Geometry check sheet. Reference: the model listing, model coordinates, mm. A direction names the side the tool comes from. Round coordinates to 2 decimals unless told otherwise and drop trailing zeros. Order: outer loops, then holes, each group sorted by start corner. A loop starts at its lowest first (then second) coordinate and runs counter-clockwise, first axis right, second up.
(1) Cross-section at A-A on x = 0. Enter the section's corners in (y, z) (1 decimal), and give its area (3 significant figures).
(2) Cross-section at B-B on z = 0. Enter the section's corners in (x, y) (1 decimal), and give its area (3 significant figures).
(3) Draft check along X on faces 3 (the face through (0, 29.21, 0)), 4 (the face through (1.93, 20.84, 2.52)), 5 (the face through (0, 3.175, 0)), 6 (the face through (-7.75, 1.57, 1.72)). Enter one of: pulls with the +X half, pulls with the -X half, needs draft (parallel to the pull), parting line crosses it, or undercut.
(4) Set-up check for faces 1 (the face through (-6, 10.16, 0)), 2 (the face through (8, 0, -2)): record each of +Z, -Z, +X, -X, +Y, -Y from which the full face is reachable in a straight line by a thin tool's end or side.
(5) Thickness scan on L1, parallel to X at y = 1.65, z = 0 (1 decimal); L2, parallel to Y at x = -2.5, z = 8.25; L3, parallel to Y at x = 5.75, z = -2 (3 decimals). Record the ranges inside material, lowest first.
(6) Cross-section at D-D on x = 7.5. Enter the section's corners in (y, z) (3 decimals), and give its area (3 significant figures).
(7) Cross-section at C-C on y = 6.5. Enter the section's corners in (x, z) (3 decimals), and give its area (3 significant figures).
(8) Gauge pin test, flat ends, axial feed: P1, Ø1.5, axis at y = 6.5, z = -2, coming from the +X side; P2, Ø5, axis at x = 3, z = 2, coming from the -Y side (3 decimals); P3, Ø6, axis at x = 3.5, y = 21.5, coming from the -Z side; P4, Ø3, axis at x = 6, y = 17.5, coming from the -Z side. Record the tip position at first contact, or that the pin passes through.
from build123d import *

# Parameters (mm, degrees)
SKETCH1_R           = 9.525
BOSS_EXTRUDE1_DEPTH = 10.16
SKETCH2_R           = 7.9375
CUT_EXTRUDE1_DEPTH  = 3.175
SKETCH3_R           = 3.175
BOSS_EXTRUDE2_DEPTH = 19.05
FILLET1_R           = 2.54


with BuildPart() as part:
    # Sketch1 → Boss-Extrude1 (new body)
    with BuildSketch(Plane(origin=(0, 0, 0), x_dir=(1, 0, 0), z_dir=(0, 1, 0))):
        with Locations(Location((0, 0, 0), (0, 0, 270))):
            Circle(SKETCH1_R)
    extrude(amount=BOSS_EXTRUDE1_DEPTH)

    # Sketch2 → Cut-Extrude1 (cut)
    with BuildSketch(Plane(origin=(0, 0, 0), x_dir=(-1, 0, 0), z_dir=(0, -1, 0))):
        with Locations(Location((0, 0, 0), (0, 0, 90))):
            Circle(SKETCH2_R)
    extrude(amount=-CUT_EXTRUDE1_DEPTH, mode=Mode.SUBTRACT)

    # Sketch3 → Boss-Extrude2 (add)
    with BuildSketch(Plane(origin=(0, 10.16, 0), x_dir=(1, 0, 0), z_dir=(0, 1, 0))):
        with Locations(Location((0, 0, 0), (0, 0, 90))):
            Circle(SKETCH3_R)
    extrude(amount=BOSS_EXTRUDE2_DEPTH)

    # Fillet1
    fillet1_edges = [part.edges().sort_by_distance(p)[0] for p in [
        (0, 10.16, 3.175),
    ]]
    fillet(fillet1_edges, radius=FILLET1_R)


solid = part.part
Found:
1. outline: (0, -9.5) - (10.2, -9.5) - (10.2, -5.7) arc R2.5 cw to (12.7, -3.2) - (29.2, -3.2) - (29.2, 3.2) - (12.7, 3.2) arc R2.5 cw to (10.2, 5.7) - (10.2, 9.5) - (0, 9.5) - (0, 7.9) - (3.2, 7.9) - (3.2, -7.9) - (0, -7.9) - close
1. area: 267 mm2
2. outline: (-9.5, 0) - (-7.9, 0) - (-7.9, 3.2) - (7.9, 3.2) - (7.9, 0) - (9.5, 0) - (9.5, 10.2) - (5.7, 10.2) arc R2.5 cw to (3.2, 12.7) - (3.2, 29.2) - (-3.2, 29.2) - (-3.2, 12.7) arc R2.5 cw to (-5.7, 10.2) - (-9.5, 10.2) - close
2. area: 267 mm2
3. face 3: needs draft
3. face 4: parting line crosses it
3. face 5: undercut
3. face 6: undercut
4. face 1: +Y
4. face 2: +Z, -Z, +X, -X, -Y
5. L1: x = -9.5 to -7.9, 7.9 to 9.5
5. L2: y = 0 to 10.16
5. L3: y = 3.175 to 10.16
6. outline: (0, -5.872) - (10.16, -5.872) - (10.16, 5.872) - (0, 5.872) - (0, 2.599) - (3.175, 2.599) - (3.175, -2.599) - (0, -2.599) - close
6. area: 103 mm2
7. outline: circle Ø19.05 at (0, 0)
7. area: 285 mm2
8. P1: stops at x = 9.44
8. P2: stops at y = 3.175
8. P3: stops at z = -3.14
8. P4: passes through
